Source: CAD feature listing. Evaluate the final solid. Frame: model axes, mm. A direction names the side the tool comes from. Give positions to 0.01 mm unless a question says otherwise; leave off trailing zeros. Write each loop counter-clockwise with the first axis right and the second up, starting at its lowest first coordinate (ties: lowest second). Pieces come first, ordered by that corner, then holes. Notation, with made-up numbers: (89.5, 89.5) -> (140.5, 89.5) arc R22 ccw to (140.5, 103.5) -> close; hole circle Ø5 at (18, 64). An arc over 180 degrees is marked (long way). Use one line per item in the form item = value. Start each with the question number.
(1) Cut plane A-A, the plane z = 3. Output: boundary loops of the cut face in (x, y).
(2) Material intervals for line 1 along X through (y, z) = (5.8, 0); line 2 along X through (y, z) = (7.25, 5.5); line 3 along X through (y, z) = (2.75, 0), sorted ascending. Write a range as from..to.
(3) Set-up query: faces 4 (the face through (44.5, 6.5, 21)), 5 (the face through (61.5, 4, 0)), 6 (the face through (30, 1, 32)), 7 (the face through (31, 3, -32)). Return all of +Z, -Z, +X, -X, +Y, -Y with unobstructed straight access to the full face (end or side cutting, diameter ignored); none if empty.
(4) Draft query along Y for faces 1 (the face through (23.505, 6.521, 0.418)), 2 (the face through (11, 5, 0)), 3 (the face through (30, 1, -32)). Return one class per face: pulls with the +Y half, pulls with the -Y half, needs draft (parallel to the pull), parting line crosses it, or undercut.
(5) First-contact query: P1, Ø0.6, axis at x = 32, y = 1.5, coming from the +Z side; P2, Ø2.5, axis at x = 30, z = 31, coming from the -Y side; P3, Ø1.6, axis at x = -55, y = 2, coming from the -Z side. Flat tips, straight axial feed; report the tip coordinate or a pass-through.
from build123d import *

# Parameters (mm, degrees)
SKETCH1_W              = 123
SKETCH1_H              = 68
BOSS_EXTRUDE1_DEPTH    = 8
CUT_EXTRUDE1_DEPTH     = 5
LPATTERN6_COUNT        = 2
LPATTERN6_PITCH        = 84
LPATTERN6_COPY_1_DEPTH = 5
SKETCH7_R              = 8
CUT_EXTRUDE2_DEPTH     = 10
SKETCH8_R              = 13
CUT_EXTRUDE3_DEPTH     = 3
CUT_EXTRUDE4_DEPTH     = 5
CUT_EXTRUDE5_DEPTH     = 3
CUT_EXTRUDE6_DEPTH     = 3
CUT_EXTRUDE7_DEPTH     = 5
FILLET2_R              = 1


with BuildPart() as part:
    # Sketch1 → Boss-Extrude1 (new body)
    with BuildSketch(Plane(origin=(0, 0, 0), x_dir=(1, 0, 0), z_dir=(0, 1, 0))):
        Rectangle(SKETCH1_W, SKETCH1_H)
    extrude(amount=BOSS_EXTRUDE1_DEPTH)

    # Sketch6 → Cut-Extrude1 (cut)
    with BuildSketch(Plane(origin=(0, 0, -34), x_dir=(-1, 0, 0), z_dir=(0, 0, -1))):
        with BuildLine():
            Line((49.5, 3), (57.5, 3))
            ThreePointArc((57.5, 3), (58.5, 2), (57.5, 1))
            Line((57.5, 1), (49.5, 1))
            ThreePointArc((49.5, 1), (48.5, 2), (49.5, 3))
        make_face()
    cut_extrude1 = extrude(amount=-CUT_EXTRUDE1_DEPTH, mode=Mode.SUBTRACT)

    # Mirror16: Cut-Extrude1 across plane
    add(cut_extrude1.mirror(Plane.XY), mode=Mode.SUBTRACT)

    # LPattern6: Cut-Extrude1 ×2
    with Locations(*[(i * LPATTERN6_PITCH, 0, 0) for i in range(1, LPATTERN6_COUNT)]):
        add(cut_extrude1, mode=Mode.SUBTRACT)

    # LPattern6 copy 1 sketch → LPattern6 copy 1 (cut)
    with BuildSketch(Plane(origin=(84, 0, 34), x_dir=(-1, 0, 0), z_dir=(0, 0, 1))):
        with BuildLine():
            Line((49.5, -3), (57.5, -3))
            ThreePointArc((57.5, -3), (58.5, -2), (57.5, -1))
            Line((57.5, -1), (49.5, -1))
            ThreePointArc((49.5, -1), (48.5, -2), (49.5, -3))
        make_face()
    extrude(amount=-LPATTERN6_COPY_1_DEPTH, mode=Mode.SUBTRACT)

    # Sketch7 → Cut-Extrude2 (cut)
    with BuildSketch(Plane(origin=(0, 8, 0), x_dir=(1, 0, 0), z_dir=(0, 1, 0))):
        with Locations(Location((-11.5, 0, 0), (0, 0, 270))):
            Circle(SKETCH7_R)
    extrude(amount=-CUT_EXTRUDE2_DEPTH, mode=Mode.SUBTRACT)

    # Sketch8 → Cut-Extrude3 (cut)
    with BuildSketch(Plane(origin=(0, 8, 0), x_dir=(1, 0, 0), z_dir=(0, 1, 0))):
        with Locations(Location((-11.5, 0, 0), (0, 0, 270))):
            Circle(SKETCH8_R)
    extrude(amount=-CUT_EXTRUDE3_DEPTH, mode=Mode.SUBTRACT)

    # Sketch9 → Cut-Extrude4 (cut)
    with BuildSketch(Plane(origin=(0, 8, 0), x_dir=(1, 0, 0), z_dir=(0, 1, 0))):
        with BuildLine():
            Line((-44.5, 8), (-44.5, -8))
            ThreePointArc((-44.5, -8), (-46.5, -10), (-48.5, -8))
            Line((-48.5, -8), (-48.5, 8))
            ThreePointArc((-48.5, 8), (-46.5, 10), (-44.5, 8))
        make_face()
    extrude(amount=-CUT_EXTRUDE4_DEPTH, mode=Mode.SUBTRACT)

    # Sketch10 → Cut-Extrude5 (cut)
    with BuildSketch(Plane(origin=(0, 8, 0), x_dir=(1, 0, 0), z_dir=(0, 1, 0))):
        with BuildLine():
            ThreePointArc((42.5, 23), (19.5, 0), (42.5, -23))
            ThreePointArc((42.5, -23), (44.5, -21), (42.5, -19))
            ThreePointArc((42.5, -19), (23.5, 0), (42.5, 19))
            ThreePointArc((42.5, 19), (44.5, 21), (42.5, 23))
        make_face()
    extrude(amount=-CUT_EXTRUDE5_DEPTH, mode=Mode.SUBTRACT)

    # Sketch11 → Cut-Extrude6 (cut)
    with BuildSketch(Plane(origin=(0, 8, 0), x_dir=(1, 0, 0), z_dir=(0, 1, 0))):
        with BuildLine():
            ThreePointArc((-11.5, -26), (14.5, 0), (-11.5, 26))
            ThreePointArc((-11.5, 26), (-13.5, 24), (-11.5, 22))
            ThreePointArc((-11.5, 22), (10.5, 0), (-11.5, -22))
            ThreePointArc((-11.5, -22), (-13.5, -24), (-11.5, -26))
        make_face()
    extrude(amount=-CUT_EXTRUDE6_DEPTH, mode=Mode.SUBTRACT)

    # Sketch12 → Cut-Extrude7 (cut)
    with BuildSketch(Plane(origin=(0, 8, 0), x_dir=(1, 0, 0), z_dir=(0, 1, 0))):
        with BuildLine():
            Line((-48.25, 3), (-44.75, 3))
            ThreePointArc((-44.75, 3), (-42.616116524, 3.883883476), (-43.5, 1.75))
            Line((-43.5, 1.75), (-43.5, -1.75))
            ThreePointArc((-43.5, -1.75), (-42.616116524, -3.883883476), (-44.75, -3))
            Line((-44.75, -3), (-48.25, -3))
            ThreePointArc((-48.25, -3), (-50.383883476, -3.883883476), (-49.5, -1.75))
            Line((-49.5, -1.75), (-49.5, 1.75))
            ThreePointArc((-49.5, 1.75), (-50.383883476, 3.883883476), (-48.25, 3))
        make_face()
    extrude(amount=-CUT_EXTRUDE7_DEPTH, mode=Mode.SUBTRACT)

    # Fillet2
    fillet2_edges = [part.edges().sort_by_distance(p)[0] for p in [
        (-48.5, 5.5, -3.75),
        (-44.5, 5.5, -3.75),
        (-44.5, 5.5, 3.75),
        (-48.5, 5.5, 3.75),
    ]]
    fillet(fillet2_edges, radius=FILLET2_R)


solid = part.part
Geometry says:
q1.outline = (-61.5, 0) -> (-18.92, 0) -> (-18.92, 5) -> (-24.15, 5) -> (-24.15, 8) -> (-42.25, 8) -> (-42.25, 3) -> (-50.75, 3) -> (-50.75, 8) -> (-61.5, 8) -> close; (-4.08, 0) -> (61.5, 0) -> (61.5, 8) -> (23.74, 8) -> (23.74, 5) -> (19.7, 5) -> (19.7, 8) -> (14.33, 8) -> (14.33, 5) -> (10.29, 5) -> (10.29, 8) -> (1.15, 8) -> (1.15, 5) -> (-4.08, 5) -> close
q2.line_1 = -61.5..-49.5, -43.5..-24.5, 1.5..10.5, 14.5..19.5, 23.5..61.5
q2.line_2 = -61.5..-48.5, -44.5..-23.28, 0.28..9.8, 13.91..20.17, 24.31..61.5
q2.line_3 = -61.5..-19.5, -3.5..61.5
q3.face_4 = +Y
q3.face_5 = +Z, -Z, +X, +Y, -Y
q3.face_6 = +Z
q3.face_7 = -Z
q4.face_1 = needs draft
q4.face_2 = pulls with the +Y half
q4.face_3 = undercut
q5.P1 = 29
q5.P2 = 0
q5.P3 = -29
